from build123d import *

# Parameters (mm, degrees)
SKETCH1_W           = 15
SKETCH1_H           = 66
SKETCH1_R           = 1.75
BOSS_EXTRUDE1_DEPTH = 10
SKETCH2_R           = 3
CUT_EXTRUDE1_DEPTH  = 6
FILLET1_R           = 2
SKETCH3_R           = 9
CUT_EXTRUDE2_DEPTH  = 15


with BuildPart() as part:
    # Sketch1 → Boss-Extrude1 (new body)
    with BuildSketch(Plane(origin=(0, 0, 0), x_dir=(1, 0, 0), z_dir=(0, 1, 0))):
        with Locations((7.5, 33)):
            Rectangle(SKETCH1_W, SKETCH1_H)
        with Locations(Location((7.5, 59.5, 0), (0, 0, 270))):
            Circle(SKETCH1_R, mode=Mode.SUBTRACT)
        with Locations(Location((7.5, 6.5, 0), (0, 0, 270))):
            Circle(SKETCH1_R, mode=Mode.SUBTRACT)
    extrude(amount=BOSS_EXTRUDE1_DEPTH)

    # Sketch2 → Cut-Extrude1 (cut)
    with BuildSketch(Plane(origin=(0, 10, 0), x_dir=(1, 0, 0), z_dir=(0, 1, 0))):
        with Locations(Location((7.5, 59.5, 0), (0, 0, 270))):
            Circle(SKETCH2_R)
        with Locations(Location((7.5, 6.5, 0), (0, 0, 270))):
            Circle(SKETCH2_R)
    extrude(amount=-CUT_EXTRUDE1_DEPTH, mode=Mode.SUBTRACT)

    # Fillet1
    fillet1_edges = [part.edges().sort_by_distance(p)[0] for p in [
        (15, 10, -33),
        (7.5, 10, -66),
        (0, 10, -33),
        (7.5, 10, 0),
    ]]
    fillet(fillet1_edges, radius=FILLET1_R)

    # Sketch3 → Cut-Extrude2 (cut)
    with BuildSketch(Plane(origin=(15, 0, 0), x_dir=(0, 0, -1), z_dir=(1, 0, 0))):
        with Locations((33, -3.75)):
            Circle(SKETCH3_R)
    extrude(amount=-CUT_EXTRUDE2_DEPTH, mode=Mode.SUBTRACT)


solid = part.part
Work out the finished part from the listing and answer in its coordinate system (mm). A direction names the side the tool comes from. Round coordinates to 2 decimals unless told otherwise and drop trailing zeros. Loops run counter-clockwise (first coordinate to the right, second up) from the corner with the lowest first, then second, coordinate; pieces in that order, holes last. Notation, with made-up numbers: (84, 11.25) - (125, 11.25) arc R16 cw to (125, 34.25) - close; hole circle Ø1 at (72, 63.5). An arc over 180 degrees is marked (long way). One line per item, written item: value.
Q1. Find section D-D on y = 7.25. Give the vertices of the cut face in (x, z), and give its area (3 significant figures).
Check values:
outline: (0, -66) - (15, -66) - (15, 0) - (0, 0) - close; hole circle Ø6 at (7.5, -59.5); hole circle Ø6 at (7.5, -6.5)
area: 933 mm2
Q2. For faces 1 (the flat face through (0, 6, -33)), 2 (the cylindrical face through (8.4, 7.04, -3.64)), determine the directions among +Z, -Z, +X, -X, +Y, -Y from which every point of the face is accessible in a straight line to the end or side of a thin tool.
Check values:
face 1: +Z, -Z, -X, +Y, -Y
face 2: +Y
Q3. Find section C-C on x = 6.5. Give the vertices of the cut face in (y, z), and give its area (3 significant figures).
Check values:
outline: (0, -66) - (8, -66) arc R2 ccw to (10, -64) - (10, -62.33) - (4, -62.33) - (4, -60.94) - (0, -60.94) - close; (0, -58.06) - (4, -58.06) - (4, -56.67) - (10, -56.67) - (10, -9.33) - (4, -9.33) - (4, -7.94) - (0, -7.94) - (0, -24.82) arc R9 cw to (0, -41.18) - close; (0, -5.06) - (4, -5.06) - (4, -3.67) - (10, -3.67) - (10, -2) arc R2 ccw to (8, 0) - (0, 0) - close
area: 506 mm2
Q4. Find section B-B on y = 2.25. Give the vertices of the cut face in (x, z).
Check values:
outline: (0, -66) - (15, -66) - (15, -39.71) - (0, -39.71) - close; (0, -26.29) - (15, -26.29) - (15, 0) - (0, 0) - close; hole circle Ø3.5 at (7.5, -59.5); hole circle Ø3.5 at (7.5, -6.5)
Q5. Straight lines are drawn through the part: probe 1 along Z at (x, y) = (8, 6.75); probe 2 along X at (y, z) = (7.6, -6.5); probe 3 along Z at (x, y) = (6.75, 3.75). For each, find the intervals that lie inside material, in ascending order.
Check values:
probe 1: -66 to -62.46, -56.54 to -9.46, -3.54 to 0
probe 2: 0 to 4.5, 10.5 to 15
probe 3: -66 to -61.08, -57.92 to -37.97, -28.03 to -8.08, -4.92 to 0
Q6. The mould has two halves that part along X. Classify faces 3 (the flat face through (6, 4, -5)), 4 (the flat face through (15, 6, -33)), 5 (the cylindrical face through (7.6, 9.4, -0.57)): +X half, -X half, draft (parallel to the pull), parting line (faces both ways), or undercut.
Check values:
face 3: undercut
face 4: +X half
face 5: draft
Q7. Find section A-A on z = -59.5. Give the vertices of the cut face in (x, y).
Check values:
outline: (0, 0) - (5.75, 0) - (5.75, 4) - (4.5, 4) - (4.5, 10) - (2, 10) arc R2 ccw to (0, 8) - close; (9.25, 0) - (15, 0) - (15, 8) arc R2 ccw to (13, 10) - (10.5, 10) - (10.5, 4) - (9.25, 4) - close
Q8. Each of these flat-tipped pins is pushed along its axis until it touches: pin 1 Ø1.8 at (x, z) = (7.5, -60.5) entering from +Y; pin 2 Ø5.5 at (x, z) = (7.5, -6.5) entering from -Y. Where does it stop, or does it pass through?
Check values:
pin 1: y = 4
pin 2: y = 0
